```python
from build123d import *

# Parameters (mm, degrees)
SKETCH1_W                      = 82
SKETCH1_H                      = 61
BOSS_EXTRUDE1_DEPTH            = 13.2
SHELL2_T                       = -1.5
SKETCH2_W                      = 7.75
SKETCH2_H                      = 7.75
BOSS_EXTRUDE2_DEPTH            = 10
BOSS_EXTRUDE3_DEPTH            = 1.7
MIRROR2_COPY_1_SKETCH_W        = 7.75
MIRROR2_COPY_1_SKETCH_H        = 7.75
MIRROR2_COPY_1_DEPTH           = 10
CUT_EXTRUDE1_REACH             = 76.674
SKETCH9_W                      = 9.5
SKETCH9_H                      = 6.7
CUT_EXTRUDE1_DIRECTION_2_DEPTH = 75.674225808


with BuildPart() as part:
    # Sketch1 → Boss-Extrude1 (new body)
    with BuildSketch(Plane(origin=(0, 0, 0), x_dir=(1, 0, 0), z_dir=(0, 1, 0))):
        Rectangle(SKETCH1_W, SKETCH1_H)
    extrude(amount=BOSS_EXTRUDE1_DEPTH)

    # Shell2
    shell2_openings = [part.faces().sort_by_distance(p)[0] for p in [
        (0, 0, 0),
    ]]
    offset(amount=SHELL2_T, openings=shell2_openings, kind=Kind.INTERSECTION)

    # Sketch2 → Boss-Extrude2 (add)
    with BuildSketch(Plane.XZ.offset(-11.7)):
        with Locations((35.625, 25.125)):
            Rectangle(SKETCH2_W, SKETCH2_H)
    boss_extrude2 = extrude(amount=BOSS_EXTRUDE2_DEPTH)

    # Mirror1: Boss-Extrude2 across plane
    add(boss_extrude2.mirror(Plane(origin=(0, 0, 0), x_dir=(0, 0, 1), z_dir=(1, 0, 0))))

    # Sketch6 → CBORE for M5 Hex Head Bolt1 (revolve, cut)
    with BuildSketch(Plane(origin=(35.25, 13.2, 25.25), x_dir=(0, 0, 1), z_dir=(1, 0, 0))):
        Polygon((0, 0), (0, 13.2), (1.375, 13.2), (1.375, 3.25), (2.75, 3.25), (2.75, 0.625), (3.375, 0), align=None)
    cbore_for_m5_hex_head_bolt1 = revolve(axis=Axis((35.25, 19.55, 25.25), (0, -1, 0)), mode=Mode.SUBTRACT)

    # Sketch8 → Boss-Extrude3 (add)
    with BuildSketch(Plane.XZ.offset(-1.7)):
        with BuildLine():
            Line((-36.35, 29), (-33.15, 29))
            ThreePointArc((-33.15, 29), (-34.75, 27.4), (-36.35, 29))
        make_face()
    boss_extrude3 = extrude(amount=BOSS_EXTRUDE3_DEPTH)

    # Mirror2: Boss-Extrude2, CBORE for M5 Hex Head Bolt1, Boss-Extrude3 across plane
    add(boss_extrude2.mirror(Plane.XY))
    add(cbore_for_m5_hex_head_bolt1.mirror(Plane.XY), mode=Mode.SUBTRACT)
    add(boss_extrude3.mirror(Plane.XY))

    # Mirror2 copy 1 sketch → Mirror2 copy 1 (add)
    with BuildSketch(Plane(origin=(0, 11.7, 0), x_dir=(-1, 0, 0), z_dir=(0, -1, 0))):
        with Locations((35.625, 25.125)):
            Rectangle(MIRROR2_COPY_1_SKETCH_W, MIRROR2_COPY_1_SKETCH_H)
    extrude(amount=MIRROR2_COPY_1_DEPTH)

    # Sketch9 → Cut-Extrude1 (cut, up to next)
    with BuildSketch(Plane.XY.offset(30.5), mode=Mode.PRIVATE) as cut_extrude1_sk1:
        with Locations((24.1, 3.35)):
            Rectangle(SKETCH9_W, SKETCH9_H)
    cut_extrude1_tool1 = extrude(cut_extrude1_sk1.sketch, amount=-CUT_EXTRUDE1_REACH, mode=Mode.PRIVATE) & part.part
    add(cut_extrude1_tool1.solids().sort_by_distance((24.1, 3.35, 30.5))[0], mode=Mode.SUBTRACT)

    # Sketch9 → Cut-Extrude1 direction 2 (cut)
    with BuildSketch(Plane.XY.offset(30.5)):
        with Locations((24.1, 3.35)):
            Rectangle(SKETCH9_W, SKETCH9_H)
    extrude(amount=CUT_EXTRUDE1_DIRECTION_2_DEPTH, mode=Mode.SUBTRACT)


solid = part.part
```
Verification items for the finished model (mm, model axes). A direction names the side the tool comes from. Coordinates: 2 decimals unless noted, no trailing zeros. Write each loop counter-clockwise with the first axis right and the second up, starting at its lowest first coordinate (ties: lowest second). Pieces come first, ordered by that corner, then holes. Notation, with made-up numbers: (-13, 65) - (12, 65) arc R26 cw to (12, 97) - close; hole circle Ø2 at (25, 84). An arc over 180 degrees is marked (long way). Write item = value, one per line.
Q1. Access from +Z, -Z, +X, -X, +Y, -Y to the whole of each face (thin tool, end or side, straight path). Record for faces 1 (the face through (34.321, 5.883, 24.237)), 2 (the face through (-1, 11.7, 0)), 3 (the face through (33.391, 11.281, -23.223)).
Answer:
face_1 = +Y, -Y
face_2 = -Y
face_3 = +Y
Q2. Mould release check, pull along X, two halves, no side actions. Record for faces 4 (the face through (37, 1.7, 25)), 5 (the face through (-1, 13.2, 0)): released by +X, released by -X, zero draft, split by the parting line, or undercut.
Answer:
face_4 = undercut
face_5 = zero draft
Q3. Cross-section at D-D (z = 15). Enter the section's corners in (x, y), plus the area to 3 significant figures.
Answer:
outline = (-41, 0) - (-39.5, 0) - (-39.5, 11.7) - (39.5, 11.7) - (39.5, 0) - (41, 0) - (41, 13.2) - (-41, 13.2) - close
area = 158 mm²
Q4. Cross-section at C-C (x = 27). Enter the section's corners in (y, z).
Answer:
outline = (0, -30.5) - (13.2, -30.5) - (13.2, 30.5) - (6.7, 30.5) - (6.7, 29) - (11.7, 29) - (11.7, -29) - (0, -29) - close
Q5. Cross-section at A-A (z = 25.25). Enter the section's corners in (x, y) (3 decimals), plus the area to 3 significant figures.
Answer:
outline = (-41, 0) - (-39.5, 0) - (-39.5, 1.7) - (-31.75, 1.7) - (-31.75, 11.7) - (31.75, 11.7) - (31.75, 1.7) - (33.875, 1.7) - (33.875, 9.95) - (32.5, 9.95) - (32.5, 12.575) - (31.875, 13.2) - (-41, 13.2) - close; (36.625, 1.7) - (39.5, 1.7) - (39.5, 0) - (41, 0) - (41, 13.2) - (38.625, 13.2) - (38, 12.575) - (38, 9.95) - (36.625, 9.95) - close
area = 272 mm²
Q6. Go/stop test with flat-tipped pins: pin 1 Ø4 at (x, z) = (33.5, -26) entering from -Y; pin 2 Ø3 at (x, z) = (35.5, 24.5) entering from +Y. Record where each tip stops, or that it passes through.
Answer:
pin_1 = 1.7
pin_2 = 9.95
Q7. Material ranges on L1, parallel to Z at x = 35.25, y = 11.1; L2, parallel to Z at x = 35.25, y = 8 (3 decimals); L3, parallel to X at y = 2.5, z = -8.5, recorded low to high. Write a range as from..to.
Answer:
L1 = -30.5..-28, -22.5..-21.25, 21.25..22.5, 28..30.5
L2 = -30.5..-26.625, -23.875..-21.25, 21.25..23.875, 26.625..30.5
L3 = -41..-39.5, 39.5..41
Q8. Cross-section at B-B (x = 35.25). Give the number of separate pieces and of enclosed holes in the cut face, plus the area to 3 significant figures.
Answer:
separate_pieces = 3
enclosed_holes = 0
area = 200 mm²
